```python
from build123d import *

# Parameters (mm, degrees)
F0_W      = 19
F0_H      = 40
F1_DEPTH  = 40
F3_DEPTH  = 25
F4_R      = 2.5
F5_DEPTH  = 25
F7_START  = -3
F6_R      = 6
F7_DEPTH  = 22
F8_R      = 2.5
F9_DEPTH  = 25
F11_START = -3
F10_R     = 6
F11_DEPTH = 22
F12_R     = 0.5


with BuildPart() as f1:
    # F0 (on Front) → F1 (new body)
    with BuildSketch(Plane.XZ):
        Rectangle(F0_W, F0_H)
    extrude(amount=F1_DEPTH)

    # F2 (on face) → F3 (cut)
    with BuildSketch(Plane.YZ.offset(9.5)):
        Polygon((0, 20), (-40, 20), (0, -20), align=None)
    extrude(amount=-F3_DEPTH, mode=Mode.SUBTRACT)

    # F4 (on face) → F5 (cut)
    with BuildSketch(Plane.XZ.offset(40)):
        with Locations((0, 7)):
            Circle(F4_R)
    extrude(amount=-F5_DEPTH, mode=Mode.SUBTRACT)

    # F6 (on face) → F7 (cut)
    with BuildSketch(Plane.XZ.offset(40).offset(F7_START)):
        with Locations((0, 7)):
            Circle(F6_R)
    extrude(amount=-F7_DEPTH, mode=Mode.SUBTRACT)

    # F8 (on face) → F9 (cut)
    with BuildSketch(Plane(origin=(0, 0, -20), x_dir=(1, 0, 0), z_dir=(0, 0, -1))):
        with Locations((0, 13)):
            Circle(F8_R)
    extrude(amount=-F9_DEPTH, mode=Mode.SUBTRACT)

    # F10 (on face) → F11 (cut)
    with BuildSketch(Plane(origin=(0, 0, -20), x_dir=(1, 0, 0), z_dir=(0, 0, -1)).offset(F11_START)):
        with Locations((0, 13)):
            Circle(F10_R)
    extrude(amount=-F11_DEPTH, mode=Mode.SUBTRACT)

    # F12
    f12_edges = [f1.edges().sort_by_distance(p)[0] for p in [
        (0, -40, 20),
        (0, 0, -20),
        (0, -40, -20),
    ]]
    fillet(f12_edges, radius=F12_R)


solid = f1.part
```
Build history of the part. All positions in model axes, mm. A direction names the side the tool comes from. Give positions to 0.01 mm unless a question says otherwise; leave off trailing zeros. Loops run counter-clockwise (first coordinate to the right, second up) from the corner with the lowest first, then second, coordinate; pieces in that order, holes last.
Item 1: Pull direction Z, two halves, no side cores. Call faces 4 (the face through (3, -37, 7)), 5 (the face through (9.5, -24, -5)), 6 (the face through (0, -10, -17)): released by +Z, released by -Z, zero draft, split by the parting line, or undercut.
Answers follow:
face 4: undercut
face 5: zero draft
face 6: released by +Z
Item 2: Slice it at D-D, the plane y = -35.5. List the corners of the cut face in (x, z), and give its area (3 significant figures).
Answers follow:
outline: (-9.5, -20) - (9.5, -20) - (9.5, 15.5) - (-9.5, 15.5) - close; hole circle Ø12 at (0, 7)
area: 561 mm2
Item 3: Slice it at A-A, the plane y = -13. List the corners of the cut face in (x, z), and give its area (3 significant figures).
Answers follow:
outline: (-9.5, -20) - (-2.5, -20) - (-2.5, -17) - (-6, -17) - (-6, -7) - (-9.5, -7) - close; (2.5, -20) - (9.5, -20) - (9.5, -7) - (6, -7) - (6, -17) - (2.5, -17) - close
area: 112 mm2
Item 4: Flat gauge pins, fed straight in: pin 1 (8 mm diameter, centred on x = 0, y = -13, fed in from +Z); pin 2 (4 mm diameter, centred on x = -3, y = -26, fed in from +Z); pin 3 (3.5 mm diameter, centred on x = -2.5, z = 4.5, fed in from +Y). Where does each tip first touch, or does it go through?
Answers follow:
pin 1: stops at z = -17
pin 2: stops at z = 3.68
pin 3: stops at y = -37
Item 5: Slice it at C-C, the plane z = 7. List the corners of the cut face in (x, y), and give its area (3 significant figures).
Answers follow:
outline: (-9.5, -40) - (-2.5, -40) - (-2.5, -37) - (-6, -37) - (-6, -27) - (-9.5, -27) - close; (2.5, -40) - (9.5, -40) - (9.5, -27) - (6, -27) - (6, -37) - (2.5, -37) - close
area: 112 mm2
Item 6: Drill centre lines: line 1 (X direction, y = -13, z = -9); line 2 (Z direction, x = 1.5, y = -15.5); line 3 (Y direction, x = 0, z = -17.7). Where is each one in solid material? Low to high.
Answers follow:
line 1: x = -9.5 to -6, 6 to 9.5
line 2: z = -20 to -17
line 3: y = -40 to -15.5, -10.5 to -2.3
Item 7: Slice it at B-B, the plane x = 0. List the corners of the cut face in (y, z).
Answers follow:
outline: (-40, -19.5) arc R0.5 ccw to (-39.5, -20) - (-15.5, -20) - (-15.5, -17) - (-19, -17) - (-19, -1) - (-21, 1) - (-37, 1) - (-37, 4.5) - (-40, 4.5) - close; (-40, 9.5) - (-37, 9.5) - (-37, 13) - (-33, 13) - (-39.15, 19.15) arc R0.5 ccw to (-40, 18.79) - close; (-10.5, -20) - (-1.21, -20) arc R0.5 ccw to (-0.85, -19.15) - (-7, -13) - (-7, -17) - (-10.5, -17) - close
Item 8: Which spindle directions (+Z, -Z, +X, -X, +Y, -Y) get a long thin tool onto all of the face, cutting with end or side? Do faces 1 (the face through (-0.78, -18.95, -10.89)), 2 (the face through (-1.301, -30.835, 1.143)), 3 (the face through (0, -20, -20)). Say none if no direction does.
Answers follow:
face 1: +Z
face 2: +Y
face 3: -Z, +X, -X, +Y, -Y
